Part model, mm, in its own coordinate system. Face numbers are marked on the shaded views. Round coordinates to 2 decimals unless told otherwise and drop trailing zeros. Loops run counter-clockwise (first coordinate to the right, second up) from the corner with the lowest first, then second, coordinate; pieces in that order, holes last. Notation, with made-up numbers: M 70,12.25 L 82,12.25 A11 cw 82,19.25 Z; hole C 30,63 d10. An arc over 180 degrees is marked long. Answer as CSV lines item,"result". Start each with the question number.
Item 1: Mould opens along Y. For the marked faces 1, 2 and 3 say: pulls with the +Y half, pulls with the -Y half, needs draft (parallel to the pull), parting line crosses it, or undercut.
Item 2: Band-saw the part on B-B (z = 5). Give the cut face in (x, y).
Item 3: Wall check: line 1 (Y direction, x = 6780.75, z = 4); line 2 (X direction, y = 3542.5, z = 3.5); line 3 (Z direction, x = 6780.5, y = 3546). Give the ranges that are in metal, low to high.
Item 4: Band-saw the part on A-A (x = 6780.25). Give the cut face in (y, z).
Item 5: Drop flat-ended pins along their axis: pin 1 Ø3.5 at (x, y) = (6783.5, 3559) entering from -Z; pin 2 Ø1.5 at (x, z) = (6777.5, 2.5) entering from -Y; pin 3 Ø1 at (x, z) = (6782, 7) entering from -Y. Give the stop position or say it passes through.
Item 6: Band-saw the part on D-D (x = 6784.5). Give the cut face in (y, z).
```python
from build123d import *

# Parameters (mm, degrees)
SKETCH1_R           = 6.35
SKETCH1_R_2         = 4.064
BOSS_EXTRUDE1_DEPTH = 5.842
SKETCH2_R           = 1.5875
BOSS_EXTRUDE2_DEPTH = 2.032


with BuildPart() as part:
    # Sketch1 → Boss-Extrude1 (new body)
    with BuildSketch(Plane.XY):
        with Locations((6780.775840345, 3542.568139787)):
            Circle(SKETCH1_R)
        with Locations((6780.775840345, 3542.568139787)):
            Circle(SKETCH1_R_2, mode=Mode.SUBTRACT)
    extrude(amount=BOSS_EXTRUDE1_DEPTH)

    # Sketch2 → Boss-Extrude2 (add)
    with BuildSketch(Plane.XY.offset(5.842)):
        with BuildLine():
            Line((6774.425840345, 3542.568139787), (6777.624987986, 3568.358977876))
            ThreePointArc((6777.624987986, 3568.358977876), (6780.775840345, 3571.143139787), (6783.926692704, 3568.358977876))
            Line((6783.926692704, 3568.358977876), (6787.125840345, 3542.568139787))
            ThreePointArc((6787.125840345, 3542.568139787), (6780.775840345, 3536.218139787), (6774.425840345, 3542.568139787))
        make_face()
        with Locations((6780.775840345, 3567.968139787)):
            Circle(SKETCH2_R, mode=Mode.SUBTRACT)
    extrude(amount=BOSS_EXTRUDE2_DEPTH)


solid = part.part
```
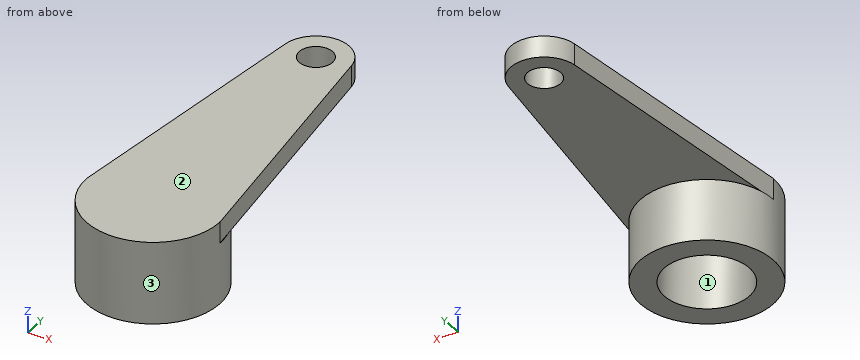
Answer block:
1,face 1,"undercut"
1,face 2,"needs draft"
1,face 3,"parting line crosses it"
2,outline,"C 6780.78,3542.57 d12.7; hole C 6780.78,3542.57 d8.13"
3,line 1,"y = 3536.22 to 3538.5, 3546.63 to 3548.92"
3,line 2,"x = 6774.43 to 6776.71, 6784.84 to 6787.13"
3,line 3,"z = 5.84 to 7.87"
4,outline,"M 3536.24,0 L 3538.54,0 L 3538.54,5.84 L 3546.6,5.84 L 3546.6,0 L 3548.9,0 L 3548.9,5.84 L 3566.47,5.84 L 3566.47,7.87 L 3536.24,7.87 Z; M 3569.47,5.84 L 3571.1,5.84 L 3571.1,7.87 L 3569.47,7.87 Z"
5,pin 1,"stops at z = 5.84"
5,pin 2,"stops at y = 3536.74"
5,pin 3,"stops at y = 3536.26"
6,outline,"M 3537.42,0 L 3540.94,0 L 3540.94,5.84 L 3544.2,5.84 L 3544.2,0 L 3547.71,0 L 3547.71,5.84 L 3563.74,5.84 L 3563.74,7.87 L 3537.42,7.87 Z"
